Can you work these out from the model? Positions are in its coordinate system, mm. Face numbers are marked on the shaded views. A direction names the side the tool comes from. Coordinates: 2 decimals unless noted, no trailing zeros. Loops run counter-clockwise (first coordinate to the right, second up) from the corner with the lowest first, then second, coordinate; pieces in that order, holes last.
```python
from build123d import *

# Parameters (mm, degrees)
SKETCH1_R           = 37.5
SKETCH1_R_2         = 10
BOSS_EXTRUDE1_DEPTH = 10
SKETCH2_R           = 40.5
SKETCH2_R_2         = 37.5
BOSS_EXTRUDE2_DEPTH = 80


with BuildPart() as part:
    # Sketch1 → Boss-Extrude1 (new body)
    with BuildSketch(Plane.XY):
        with BuildLine():
            Line((-79.8125, 21.10011478), (-16.493055556, 44.544686759))
            ThreePointArc((-16.493055556, 44.544686759), (-0.350796057, 47.498704636), (15.833333333, 44.783429475))
            Line((15.833333333, 44.783429475), (82.5, 21.213203436))
            ThreePointArc((82.5, 21.213203436), (97.448185953, -1.526088923), (79.56, -22.033075137))
            Line((79.56, -22.033075137), (15.970417375, -44.734726655))
            ThreePointArc((15.970417375, -44.734726655), (-0.27805837, -47.499186136), (-16.493055556, -44.544686759))
            Line((-16.493055556, -44.544686759), (-79.8125, -21.10011478))
            ThreePointArc((-79.8125, -21.10011478), (-94.5, 0), (-79.8125, 21.10011478))
        make_face()
        Circle(SKETCH1_R, mode=Mode.SUBTRACT)
        with Locations((-72, 0)):
            Circle(SKETCH1_R_2, mode=Mode.SUBTRACT)
        with Locations((75, 0)):
            Circle(SKETCH1_R_2, mode=Mode.SUBTRACT)
    extrude(amount=BOSS_EXTRUDE1_DEPTH)

    # Sketch2 → Boss-Extrude2 (add)
    with BuildSketch(Plane.XY.offset(10)):
        Circle(SKETCH2_R)
        Circle(SKETCH2_R_2, mode=Mode.SUBTRACT)
    extrude(amount=BOSS_EXTRUDE2_DEPTH)


solid = part.part
```
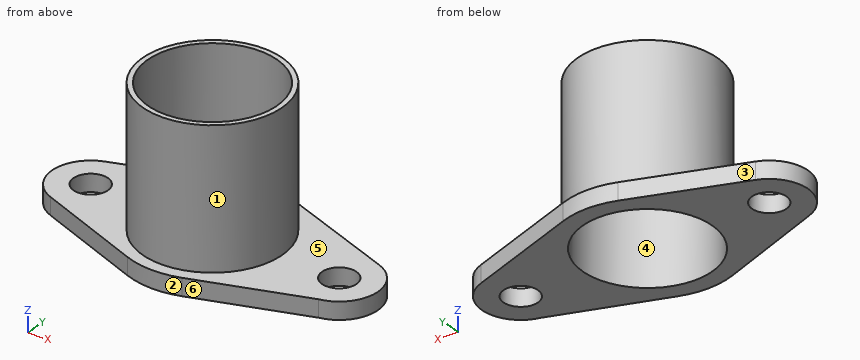
(1) I'm going to push flat-ended pins straight in: pin 1 (18 mm diameter, centred on x = 75, y = 0, fed in from +Z); pin 2 (4 mm diameter, centred on y = 7, z = 73, fed in from -X); pin 3 (3 mm diameter, centred on x = 69, z = 10, fed in from +Y); pin 4 (8 mm diameter, centred on x = 30, z = 16, fed in from +Y). Where does each tip first touch, or does it pass through?
Check values:
pin 1: passes through
pin 2: stops at x = -40.19
pin 3: stops at y = 26.52
pin 4: stops at y = 31.05
(2) I want a section at D-D on z = 81. Write out the boundary of the cut face in (x, y), then the cut area to 3 significant figures.
Check values:
outline: circle Ø81 at (0, 0); hole circle Ø75 at (0, 0)
area: 735 mm2
(3) I want a section at A-A on y = 0. Write out the boundary of the cut face in (x, z), then the cut area to 3 significant figures.
Check values:
outline: (-94.5, 0) - (-82, 0) - (-82, 10) - (-94.5, 10) - close; (-62, 0) - (-37.5, 0) - (-37.5, 90) - (-40.5, 90) - (-40.5, 10) - (-62, 10) - close; (37.5, 0) - (65, 0) - (65, 10) - (40.5, 10) - (40.5, 90) - (37.5, 90) - close; (85, 0) - (97.5, 0) - (97.5, 10) - (85, 10) - close
area: 1,250 mm2
(4) Which directions (+Z, -Z, +X, -X, +Y, -Y) give clear straight access to the entire face, cutting with the end or side of a thin tool? Please do the marked faces 5 and 6.
Check values:
face 5: +Z
face 6: +Z, -Z, +X, -Y
(5) I want a section at B-B on x = 0. Write out the boundary of the cut face in (y, z), then the cut area to 3 significant figures.
Check values:
outline: (-47.5, 0) - (-37.5, 0) - (-37.5, 90) - (-40.5, 90) - (-40.5, 10) - (-47.5, 10) - close; (37.5, 0) - (47.5, 0) - (47.5, 10) - (40.5, 10) - (40.5, 90) - (37.5, 90) - close
area: 680 mm2
(6) If I drill on probe 1 along Z at (x, y) = (81, 13.5); probe 2 along Y at (x, z) = (34, 7); probe 3 along X at (y, z) = (30, 51), over which ranges is the centre line in solid material (lowest first)?
Check values:
probe 1: z = 0 to 10
probe 2: y = -38.3 to -15.82, 15.82 to 38.36
probe 3: x = -27.21 to -22.5, 22.5 to 27.21
(7) I want a section at C-C on y = -15. Write out the boundary of the cut face in (x, z).
Check values:
outline: (-88.77, 0) - (-34.37, 0) - (-34.37, 90) - (-37.62, 90) - (-37.62, 10) - (-88.77, 10) - close; (34.37, 0) - (91.77, 0) - (91.77, 10) - (37.62, 10) - (37.62, 90) - (34.37, 90) - close
(8) If we mould it in two halves opening along Y, with no side actions, what happens to the marked faces 1, 2, 3 and 4? For each: released by +Y, released by -Y, zero draft, split by the parting line, or undercut.
Check values:
face 1: split by the parting line
face 2: released by -Y
face 3: released by +Y
face 4: undercut
